For this review, take the finished solid that the model builds, in its own axes (mm). Face numbers are marked on the shaded views. A direction names the side the tool comes from. Give positions to 0.01 mm unless a question says otherwise; leave off trailing zeros. Write each loop counter-clockwise with the first axis right and the second up, starting at its lowest first coordinate (ties: lowest second). Pieces come first, ordered by that corner, then holes. Notation, with made-up numbers: M -23,-12.5 L 11,-12.5 A37 cw 11,26.5 Z; hole C 16,22 d7. An arc over 180 degrees is marked long. One line per item, written item: value. Start each with the question number.
Item 1: Mouldability with a two-part tool opening along X and no side actions: class the marked faces 1, 2, 3 and 4 as released by +X, released by -X, zero draft, split by the parting line, or undercut.
Item 2: Consider section D-D, the plane z = -20.9. Write out the cut boundary in (x, y), and give its area (3 significant figures).
Item 3: To check wall thickness, follow probe 1 along X at (y, z) = (1.5, -29); probe 2 along X at (y, z) = (9.25, -29); probe 3 along X at (y, z) = (10, -28). State the ranges of each line that lie inside material, in increasing order.
Item 4: Consider section A-A, the plane x = 7. Write out the cut boundary in (y, z), and give its area (3 significant figures).
Item 5: Clearance check with flat-ended pins moving along their axes: pin 1 Ø4 at (y, z) = (2.5, -24) entering from +X; pin 2 Ø5.5 at (x, z) = (13, -30) entering from +Y; pin 3 Ø1.9 at (y, z) = (5.5, -20.5) entering from -X. State where each tip first meets the part, or that it passes through.
Item 6: Consider section B-B, the plane z = -29. Give the number of separate pieces and of enclosed holes in the cut face, and give its area (3 significant figures).
Item 7: Tool access review of the marked faces 5 and 6: name each direction out of +Z, -Z, +X, -X, +Y, -Y from which nothing blocks a thin tool from reaching the whole face with its end or side.
Autodesk Inventor part; units mm, degrees
ref_plane "YZ Plane" through (0, 0, 0) normal (1, 0, 0) x (0, 1, 0)
ref_plane "XZ Plane" through (0, 0, 0) normal (0, 1, 0) x (-1, 0, 0)
ref_plane "XY Plane" through (0, 0, 0) normal (0, 0, 1) x (1, 0, 0)
sketch "Sketch1" plane through (0, 0, 0) normal (0, 1, 0) x (-1, 0, 0)
  line L0 (0, 0) -> (-27, 0)
  line L1 (-27, 0) -> (-27, -33)
  line L2 (-27, -33) -> (0, -33)
  line L3 (0, -33) -> (0, 0)
  dimension "d0" = 33
  dimension "d1" = 27
extrude "Extrusion1" add sketch "Sketch1" along normal blind 11.5
sketch "Sketch2" plane through (0, 0, -33) normal (-1, 0, 0) x (0, 0, 1)
  circle A0 centre (27.25, 5.75) radius 3.5
  line L0 (0, 11.5) -> (33, 11.5)
  line L1 (33, 0) -> (33, 11.5)
  dimension "d4" = 7
  dimension "d5" = 5.75
  dimension "d6" = 5.75
extrude "Extrusion2" add sketch "Sketch2" along normal blind 5
sketch "Sketch3" plane through (0, 11.5, 0) normal (0, 1, 0) x (1, 0, 0)
  line L0 (27, 33) -> (0, 33)
  line L1 (9, 33) -> (18, 33)
  line L2 (18, 33) -> (18, 26)
  line L3 (18, 26) -> (9, 26)
  line L4 (9, 26) -> (9, 33)
  line L5 (27, 0) -> (27, 33)
  point P0 (0, 0)
  dimension "d9" = 9
  dimension "d10" = 9
  dimension "d11" = 7
extrude "Extrusion3" cut sketch "Sketch3" against normal blind 9
sketch "Sketch4" plane through (0, 11.5, 0) normal (0, 1, 0) x (1, 0, 0)
  circle A0 centre (5.5, 29) radius 2.5
  circle A1 centre (21.5, 29) radius 2.5
  line L0 (9, 33) -> (18, 33) construction
  line L1 (13.5, 33) -> (13.5, 0) construction
  line L2 (0, 0) -> (27, 0) construction
  line L3 (9, 33) -> (0, 33) construction
  dimension "d14" = 5
  dimension "d15" = 5
  dimension "d16" = 16
  dimension "d17" = 8
  dimension "d18" = 4
  dimension "d19" = 8
extrude "Extrusion4" cut sketch "Sketch4" against normal blind 15
sketch "Sketch5" plane through (0, 0, -33) normal (-1, 0, 0) x (0, 0, 1)
  circle A0 centre (4, 5.75) radius 2.05
  line L0 (0, 0) -> (0, 11.5)
  line L1 (33, 0) -> (33, 11.5) construction
  line L2 (33, 5.75) -> (0, 5.75) construction
  dimension "d22" = 4.1
  dimension "d23" = 4
  dimension "d24" = 0
extrude "Extrusion5" cut sketch "Sketch5" against normal blind 31.75
sketch "Sketch6" plane through (0, 0, 0) normal (0, -1, 0) x (1, 0, 0)
  point P0 (0, 0)
sketch "Sketch12" plane through (27, 0, -33) normal (1, 0, 0) x (0, 0, -1)
  line L0 (-33, 0) -> (0, 0)
  line L1 (-8.9949, 0) -> (-8.9949, 11.5163)
  point P0 (-32.75, 0)
sketch "Sketch13" plane through (0, 0, -33) normal (-1, 0, 0) x (0, 0, 1)
  line L0 (0, 0) -> (33, 0)
  line L1 (9, 0) -> (9, 11.5008)
  point P0 (32.75, 0)
sketch "Sketch16" plane through (0, 11.5, 0) normal (0, 1, 0) x (1, 0, 0)
  line L0 (0, 33) -> (0, 0)
  line L1 (27, 0) -> (27, 33)
  line L2 (11, 24) -> (11, 0)
  line L3 (21, 0) -> (21, 24)
  line L4 (0, 24) -> (11, 24)
  line L5 (21, 24) -> (27, 24)
sketch "Sketch17" plane through (0, 0, 0) normal (0, 0, 1) x (1, 0, 0)
  line L0 (0, 11.5) -> (27, 11.5)
  line L1 (11, 11.5) -> (11, 0)
  line L2 (21, 0) -> (21, 11.5)
  point P0 (0, 0)
sketch "Sketch18" plane through (0, 0, 0) normal (0, -1, 0) x (1, 0, 0)
  line L0 (27, 0) -> (27, -33)
  line L1 (0, 0) -> (27, 0)
  line L2 (21, 0) -> (21, -24)
  line L3 (11, 0) -> (11, -24)
  line L4 (27, -24) -> (21, -24)
  line L5 (11, -24) -> (0, -24)
  line L6 (27, -24) -> (27, -33)
  line L7 (0, -33) -> (0, 0)
  line L8 (0, -24) -> (0, -33)
  line L9 (0, -33) -> (27, -33)
  line L10 (21, 0) -> (11, 0)
fillet "Fillet5" radius 0.2 1 edges at (13.5, 11.5, 0)
fillet "Fillet7" radius 0.2 4 edges at (4.5, 11.5, -33) (22.5, 11.5, -33) (13.5, 0, -33) (13.5, 0, 0)
sketch "Sketch20" plane through (9, 2.5, -26) normal (1, 0, 0) x (0, 0, -1)
  line L0 (0, 6) -> (7, 6)
  line L1 (7, 8.8) -> (7, 0)
  line L2 (0, 6) -> (7, 6) construction
  line L3 (0, 9) -> (6.8, 9)
  line L4 (5.2368, 1.5) -> (10, 1.5) construction
  line L5 (0, 1.5) -> (0, 6)
  line L6 (0, 9) -> (0, 0)
  line L7 (0, 0) -> (0, 1)
  line L8 (0, 1) -> (5.2368, 1)
  line L9 (7, 6) -> (5.5, 6)
  line L10 (5.5, 6) -> (5.5, 1)
  line L11 (5.5, 1) -> (5.2368, 1)
  point P0 (-26, -2.5)
  dimension "d41" = 0
  dimension "d43" = 1
  dimension "d44" = 1.5
extrude "Extrusion6" cut sketch "Sketch20" against normal blind 3
sketch "Sketch21" plane through (18, 2.5, -26) normal (-1, 0, 0) x (0, 0, 1)
  line L0 (-7, 0) -> (0, 0)
  line L1 (0, 0) -> (0, 1)
  line L2 (0, 9) -> (0, 0)
  line L3 (0, 1) -> (-5.5, 1)
  line L4 (0, 9) -> (0, 6)
  line L5 (0, 6) -> (-5.5, 6)
  line L6 (-5.5, 6) -> (-5.5, 1)
  point P0 (26, -2.5)
  dimension "d47" = 1
  dimension "d48" = 5.5
  dimension "d49" = 3
  dimension "d50" = 5.5
extrude "Extrusion7" cut sketch "Sketch21" against normal blind 3
sketch "Sketch22" plane through (0, 0, -32.8) normal (-1, 0, 0) x (0, 0, 1)
  point P0 (32.8, 0)
sketch "Sketch23" plane through (0, 0, -32.8) normal (-1, 0, 0) x (0, 0, 1)
  line L0 (32.8, 0.2) -> (32.8, 11.3)
  line L1 (32.8, 5.75) -> (56.8, 5.75) construction
  circle A0 centre (11.9, 5.75) radius 1.9
  point P0 (32.8, 0)
extrude "Extrusion8" add sketch "Sketch23" along normal blind 1
sketch "Sketch24" plane through (27, 0, -0.2) normal (1, 0, 0) x (0, 0, -1)
  line L0 (-0.2, 0.2) -> (-0.2, 11.3)
  circle A0 centre (20.7, 5.75) radius 1.9
  circle A1 centre (5.9, 5.75) radius 1.9
  point P0 (-0.2, 0)
extrude "Extrusion9" add sketch "Sketch24" along normal blind 1
properties part number "MS 1.5A Servo"
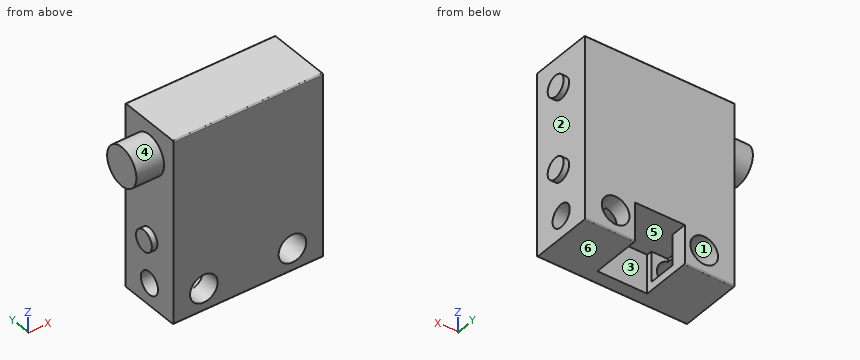
Model answer:
1. face 1: undercut
1. face 2: released by +X
1. face 3: undercut
1. face 4: zero draft
2. outline: M -1,3.85 L 0,3.85 L 0,0 L 27,0 L 27,3.85 L 28,3.85 L 28,7.65 L 27,7.65 L 27,11.5 L 0,11.5 L 0,7.65 L -1,7.65 Z
2. area: 318 mm2
3. probe 1: x = 0 to 3, 8 to 19, 24 to 27
3. probe 2: x = 0 to 3, 8 to 9, 18 to 19, 24 to 27
3. probe 3: x = 0 to 3.21, 7.79 to 9, 18 to 19.21, 23.79 to 27
4. outline: M 0,-32.8 A0.2 ccw 0.2,-33 L 11.3,-33 A0.2 ccw 11.5,-32.8 L 11.5,-31 L 8.5,-31 L 8.5,-31.5 L 3.5,-31.5 L 3.5,-31 L 0,-31 Z; M 0,-27 L 3.5,-27 L 3.5,-26 L 8.5,-26 L 8.5,-27 L 11.5,-27 L 11.5,-0.2 A0.2 ccw 11.3,0 L 0.2,0 A0.2 ccw 0,-0.2 Z
4. area: 326 mm2
5. pin 1: stops at x = 27
5. pin 2: stops at y = 2.5
5. pin 3: stops at x = -1
6. separate pieces: 7
6. enclosed holes: 0
6. area: 79.9 mm2
7. face 5: none
7. face 6: -Z, +X, -X, +Y, -Y
